Verification items for the finished model (mm, model axes). A direction names the side the tool comes from. Round coordinates to 2 decimals unless told otherwise and drop trailing zeros. Write each loop counter-clockwise with the first axis right and the second up, starting at its lowest first coordinate (ties: lowest second). Pieces come first, ordered by that corner, then holes. Notation, with made-up numbers: (11.5, 83.25) - (49.5, 83.25) arc R12 ccw to (49.5, 100.25) - close; hole circle Ø3 at (-23, -15.5). An arc over 180 degrees is marked (long way). Answer as a JSON object with one key per item and string values. Group by question number.
1) Mould release check, pull along Z, two halves, no side actions. Record for faces 1 (the flat face through (-1, -3, -58.547)), 2 (the flat face through (-58.547, -3, 1)), 3 (the flat face through (5.994, -3, 0)): +Z half, -Z half, draft (parallel to the pull), parting line (faces both ways), or undercut.
2) Thickness scan on line 1 (X direction, y = -3, z = 27); line 2 (Z direction, x = 24.5, y = -1.25); line 3 (Z direction, x = -7, y = -1.25). Record the ranges inside material, lowest first.
3) Section check B-B (x = -19). Enter the section's corners in (y, z).
4) Section check C-C (y = -5.25). Enter the section's corners in (x, z) (3 decimals), then the cut area to 3 significant figures.
5) Section check A-A (z = -28). Enter the section's corners in (x, y), then the cut area to 3 significant figures.
6) Set-up check for faces 4 (the flat face through (1, -3, 58.547)), 5 (the cylindrical face through (38.3, -3.2, 32.5)): record each of +Z, -Z, +X, -X, +Y, -Y from which the full face is reachable in a straight line by a thin tool's end or side.
```python
from build123d import *

# Parameters (mm, degrees)
F0_R     = 1.6002
F1_DEPTH = 6.35
F2_R     = 2.54


with BuildPart() as f1:
    # F0 (on Front) → F1 (new body)
    with BuildSketch(Plane.XZ):
        Polygon((58.547, 58.547), (0, 58.547), (-58.547, 58.547), (-58.547, 0), (-58.547, -58.547), (0, -58.547), (58.547, -58.547), (58.547, 0), align=None)
        with Locations((-22.5044, -47.625)):
            Circle(F0_R, mode=Mode.SUBTRACT)
        with Locations((22.5044, -47.625)):
            Circle(F0_R, mode=Mode.SUBTRACT)
        Polygon((-39.0144, 33.274), (-5.9944, 33.274), (-5.9944, 0), (-5.9944, -33.274), (-39.0144, -33.274), (-39.0144, 0), align=None, mode=Mode.SUBTRACT)
        with Locations((-22.5044, 47.625)):
            Circle(F0_R, mode=Mode.SUBTRACT)
        Polygon((5.9944, 0), (5.9944, 33.274), (39.0144, 33.274), (39.0144, 0), (39.0144, -33.274), (5.9944, -33.274), align=None, mode=Mode.SUBTRACT)
        with Locations((22.5044, 47.625)):
            Circle(F0_R, mode=Mode.SUBTRACT)
    extrude(amount=F1_DEPTH)

    # F2
    f2_edges = [f1.edges().sort_by_distance(p)[0] for p in [
        (39.0144, -3.175, 33.274),
        (39.0144, -3.175, -33.274),
        (-5.9944, -3.175, -33.274),
        (-5.9944, -3.175, 33.274),
        (5.9944, -3.175, 33.274),
        (-39.0144, -3.175, 33.274),
        (5.9944, -3.175, -33.274),
        (-39.0144, -3.175, -33.274),
    ]]
    fillet(f2_edges, radius=F2_R)


solid = f1.part
```
Returned:
{
 "1": {"face 1": "-Z half", "face 2": "draft", "face 3": "undercut"},
 "2": {"line 1": "-58.55 to -39.01, -5.99 to 5.99, 39.01 to 58.55", "line 2": "-58.55 to -33.27, 33.27 to 58.55", "line 3": "-58.55 to -32.76, 32.76 to 58.55"},
 "3": {"outline": "(-6.35, -58.55) - (0, -58.55) - (0, -33.27) - (-6.35, -33.27) - close; (-6.35, 33.27) - (0, 33.27) - (0, 58.55) - (-6.35, 58.55) - close"},
 "4": {"outline": "(-58.547, -58.547) - (58.547, -58.547) - (58.547, 58.547) - (-58.547, 58.547) - close; hole (-39.014, -30.734) arc R2.54 ccw to (-36.474, -33.274) - (-8.534, -33.274) arc R2.54 ccw to (-5.994, -30.734) - (-5.994, 30.734) arc R2.54 ccw to (-8.534, 33.274) - (-36.474, 33.274) arc R2.54 ccw to (-39.014, 30.734) - close; hole circle Ø3.2 at (-22.504, -47.625); hole circle Ø3.2 at (-22.504, 47.625); hole (5.994, -30.734) arc R2.54 ccw to (8.534, -33.274) - (36.474, -33.274) arc R2.54 ccw to (39.014, -30.734) - (39.014, 30.734) arc R2.54 ccw to (36.474, 33.274) - (8.534, 33.274) arc R2.54 ccw to (5.994, 30.734) - close; hole circle Ø3.2 at (22.504, -47.625); hole circle Ø3.2 at (22.504, 47.625)", "area": "9,300 mm2"},
 "5": {"outline": "(-58.55, -6.35) - (-39.01, -6.35) - (-39.01, 0) - (-58.55, 0) - close; (-5.99, -6.35) - (5.99, -6.35) - (5.99, 0) - (-5.99, 0) - close; (39.01, -6.35) - (58.55, -6.35) - (58.55, 0) - (39.01, 0) - close", "area": "324 mm2"},
 "6": {"face 4": "+Z, +X, -X, +Y, -Y", "face 5": "+Y, -Y"}
}
